Build history of the part. All positions in model axes, mm. Round coordinates to 2 decimals unless told otherwise and drop trailing zeros. Write each loop counter-clockwise with the first axis right and the second up, starting at its lowest first coordinate (ties: lowest second). Pieces come first, ordered by that corner, then holes. Notation, with made-up numbers: (21.5, 11.25) - (26.5, 11.25) arc R12 ccw to (26.5, 27.25) - close; hole circle Ø1 at (42, 57.5). An arc over 180 degrees is marked (long way). Answer as a JSON object with one key per item and string values. Group by question number.
Item 1: Flat gauge pins, fed straight in: pin 1 (6 mm diameter, centred on x = 5, z = 26, fed in from +Y); pin 2 (12 mm diameter, centred on x = -27.5, y = -22, fed in from +Z); pin 3 (3 mm diameter, centred on x = 5.5, y = -7.5, fed in from +Z); pin 4 (1 mm diameter, centred on x = -15, y = -5, fed in from +Z). Where does each tip first touch, or does it go through?
Item 2: Slice it at B-B, the plane x = 21.5. List the corners of the cut face in (y, z), then the cut area to 3 significant figures.
Item 3: Probe line 1 (X direction, y = -19.25, z = 37); line 2 (X direction, y = -12.75, z = 51); line 3 (Z direction, x = -9, y = -19.5). List the from-to ranges inside material, lowest first. Write a range as from..to.
Item 4: Slice it at C-C, the plane z = 46. List the corners of the cut face in (x, y), then the cut area to 3 significant figures.
Item 5: Slice it at A-A, the plane y = -16.25. List the corners of the cut face in (x, z).
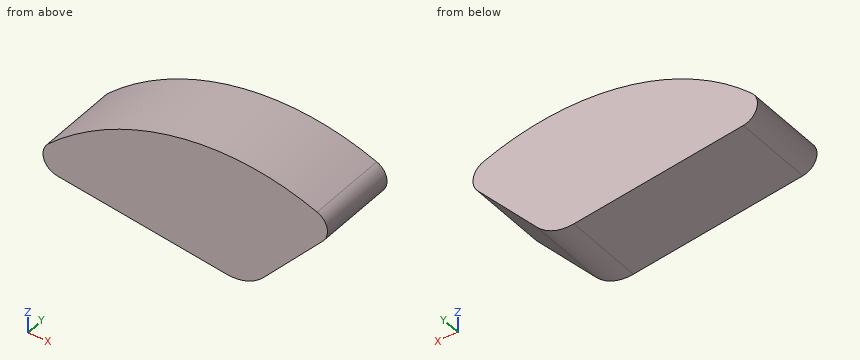
from build123d import *

# Parameters (mm, degrees)
F1_DEPTH = 25.4
F2_R     = 5.08


with BuildPart() as f1:
    # F0 (on Front) → F1 (new body)
    with BuildSketch(Plane.XZ):
        with BuildLine():
            Line((14.329544, 25.6199), (37.121165, 49.801257))
            ThreePointArc((37.121165, 49.801257), (-13.598421, 57.291577), (-57.827495, 31.361472))
            Line((-57.827495, 31.361472), (3.116123, 21.784617))
            ThreePointArc((3.116123, 21.784617), (9.197626, 22.314083), (14.329544, 25.6199))
        make_face()
    extrude(amount=F1_DEPTH)

    # F2
    f2_edges = [f1.edges().sort_by_distance(p)[0] for p in [
        (-57.827495, -12.7, 31.361472),
        (37.121165, -12.7, 49.801257),
    ]]
    fillet(f2_edges, radius=F2_R)


solid = f1.part
Geometry says:
{
 "1": {"pin 1": "stops at y = 0", "pin 2": "stops at z = 55.32", "pin 3": "stops at z = 58.65", "pin 4": "stops at z = 57.11"},
 "2": {"outline": "(-25.4, 33.23) - (0, 33.23) - (0, 55.97) - (-25.4, 55.97) - close", "area": "578 mm^2"},
 "3": {"line 1": "x = -52.01..25.06", "line 2": "x = -32.51..32.84", "line 3": "z = 23.69..58.04"},
 "4": {"outline": "(-41.31, -25.4) - (33.2, -25.4) - (33.2, 0) - (-41.31, 0) - close", "area": "1,890 mm^2"},
 "5": {"outline": "(-50.82, 38.62) arc R5.08 ccw to (-48.19, 29.85) - (3.12, 21.78) arc R12.7 ccw to (14.33, 25.62) - (32.31, 44.7) arc R5.08 ccw to (30.55, 52.88) arc R77.21 ccw to start"}
}
